```python
from build123d import *

# Parameters (mm, degrees)
BOSS_EXTRUDE1_DEPTH = 5
SHELL1_T            = -1.5


with BuildPart() as part:
    # Sketch1 → Boss-Extrude1 (new body)
    with BuildSketch(Plane.XY):
        Polygon((6.226497308, -22.124355653), (9, -17.320508076), (9, 17.320508076), (6.226497308, 22.124355653), (-6.226497308, 22.124355653), (-9, 17.320508076), (-9, -17.320508076), (-6.226497308, -22.124355653), align=None)
    extrude(amount=-BOSS_EXTRUDE1_DEPTH)

    # Shell1
    shell1_openings = [part.faces().sort_by_distance(p)[0] for p in [
        (0, 0, -5),
    ]]
    offset(amount=SHELL1_T, openings=shell1_openings, kind=Kind.INTERSECTION)


solid = part.part
```
CAD build for the part. Positions are in the model's coordinates, mm. A direction names the side the tool comes from. Give positions to 0.01 mm unless a question says otherwise; leave off trailing zeros. Order: outer loops, then holes, each group sorted by start corner. A loop starts at its lowest first (then second) coordinate and runs counter-clockwise, first axis right, second up.
(1) Saw through at A-A, the plane z = -2.55. Give the cut face in (x, y), then the cut area to 3 significant figures.
(2) Drill centre lines: L1, parallel to X at y = 8, z = -3.3; L2, parallel to Y at x = 0.75, z = -1.7; L3, parallel to Z at x = -5.5, y = -2.5. Where is each one in solid material? Low to high.
(3) Flat gauge pin, fed straight in: pin 1 (5 mm diameter, centred on x = 1.5, y = -16, fed in from -Z). Where does the tip first touch, or does it go through?
(4) Saw through at C-C, the plane y = -4. Give the cut face in (x, z).
(5) Saw through at B-B, the plane x = -2.75. Give the cut face in (y, z), then the cut area to 3 significant figures.
(6) Mould opens along X. For faces 3 (the flat face through (0, 22.124, -2)), 4 (the flat face through (-7.59, 19.76, -2.46)), 5 (the flat face through (6.445, 18.746, -3.226)), 6 (the flat face through (9, 0, -2)) say: released by +X, released by -X, zero draft, split by the parting line, or undercut.
(7) Tool access for faces 1 (the flat face through (0, 0, -1.5)), 2 (the flat face through (0, -22.124, -2)): list every direction of +Z, -Z, +X, -X, +Y, -Y with a clear straight run to the whole face (end or side of a thin tool).
Results found:
1. outline: (-9, -17.32) - (-6.23, -22.12) - (6.23, -22.12) - (9, -17.32) - (9, 17.32) - (6.23, 22.12) - (-6.23, 22.12) - (-9, 17.32) - close; hole (-7.5, -16.92) - (-5.36, -20.62) - (5.36, -20.62) - (7.5, -16.92) - (7.5, 16.92) - (5.36, 20.62) - (-5.36, 20.62) - (-7.5, 16.92) - close
1. area: 167 mm2
2. L1: x = -9 to -7.5, 7.5 to 9
2. L2: y = -22.12 to -20.62, 20.62 to 22.12
2. L3: z = -1.5 to 0
3. pin 1: stops at z = -1.5
4. outline: (-9, -5) - (-7.5, -5) - (-7.5, -1.5) - (7.5, -1.5) - (7.5, -5) - (9, -5) - (9, 0) - (-9, 0) - close
5. outline: (-22.12, -5) - (-20.62, -5) - (-20.62, -1.5) - (20.62, -1.5) - (20.62, -5) - (22.12, -5) - (22.12, 0) - (-22.12, 0) - close
5. area: 76.9 mm2
6. face 3: zero draft
6. face 4: released by -X
6. face 5: undercut
6. face 6: released by +X
7. face 1: -Z
7. face 2: +Z, -Z, +X, -X, -Y
